Work out the finished part from the listing and answer in its coordinate system (mm). Coordinates: 2 decimals unless noted, no trailing zeros. Order: outer loops, then holes, each group sorted by start corner. A loop starts at its lowest first (then second) coordinate and runs counter-clockwise, first axis right, second up.
1. The part is cut by section B-B, the plane y = -40. Give the vertices of the cut face in (x, z).
2. Find the intervals of material crossed by probe 1 along X at (y, z) = (45.5, 1.7); probe 2 along Y at (x, z) = (59.5, 0.75), in increasing order.
3. The part is cut by section C-C, the plane x = -14. Give the vertices of the cut face in (y, z).
4. The part is cut by section A-A, the plane z = 0.7. Give the vertices of the cut face in (x, y), then the cut area to 3 significant figures.
```python
from build123d import *

# Parameters (mm, degrees)
F0_W     = 355.619341
F0_H     = 250.18812
F0_W_2   = 200
F0_H_2   = 200
F1_DEPTH = 3


with BuildPart() as f1:
    # F0 (on Top) → F1 (new body)
    with BuildSketch(Plane.XY):
        with Locations((17.476574, -10.373693)):
            Rectangle(F0_W, F0_H)
        Rectangle(F0_W_2, F0_H_2, mode=Mode.SUBTRACT)
    extrude(amount=F1_DEPTH)


solid = f1.part
```
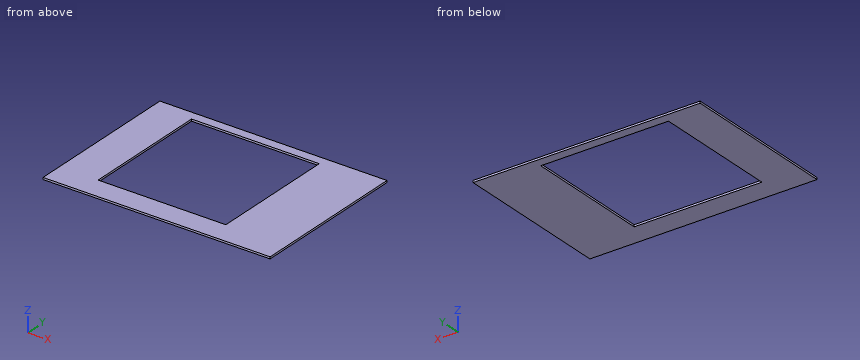
Geometry says:
1. outline: (-160.33, 0) - (-100, 0) - (-100, 3) - (-160.33, 3) - close; (100, 0) - (195.29, 0) - (195.29, 3) - (100, 3) - close
2. probe 1: x = -160.33 to -100, 100 to 195.29
2. probe 2: y = -135.47 to -100, 100 to 114.72
3. outline: (-135.47, 0) - (-100, 0) - (-100, 3) - (-135.47, 3) - close; (100, 0) - (114.72, 0) - (114.72, 3) - (100, 3) - close
4. outline: (-160.33, -135.47) - (195.29, -135.47) - (195.29, 114.72) - (-160.33, 114.72) - close; hole (-100, -100) - (100, -100) - (100, 100) - (-100, 100) - close
4. area: 49,000 mm2
